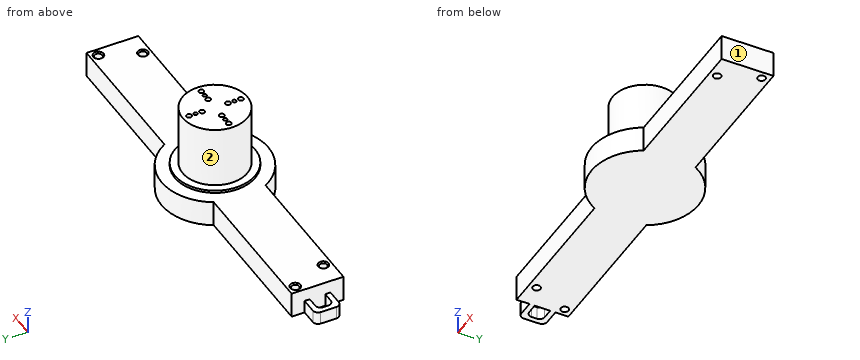
from build123d import *

# Parameters (mm, degrees)
SZKIC1_W                    = 150
SZKIC1_H                    = 20
DODANIE_WYCI_GNI_CIE1_DEPTH = 10
SZKIC2_R                    = 20.61119484
DODANIE_WYCI_GNI_CIE2_DEPTH = 10
SZKIC3_R                    = 12.5
DODANIE_WYCI_GNI_CIE5_DEPTH = 25
SZKIC8_R                    = 15.5
DODANIE_WYCI_GNI_CIE6_DEPTH = 1
SZKIC9_R                    = 1.5
WYTNIJ_WYCI_GNI_CIE1_DEPTH  = 10
SFAZOWANIE1_SIZE            = 0.5
SZKIC10_W                   = 5
SZKIC10_H                   = 10
DODANIE_WYCI_GNI_CIE7_DEPTH = 8
SZKIC11_W                   = 6
SZKIC11_H                   = 6
WYTNIJ_WYCI_GNI_CIE2_DEPTH  = 8
ZAOKR_GLENIE1_R             = 2
SZKIC12_R                   = 1
SZKIC12_R_2                 = 0.75
WYTNIJ_WYCI_GNI_CIE3_DEPTH  = 5


with BuildPart() as part:
    # Szkic1 → Dodanie-wyciągnięcie1 (new body)
    with BuildSketch(Plane.XY):
        Rectangle(SZKIC1_W, SZKIC1_H)
    extrude(amount=DODANIE_WYCI_GNI_CIE1_DEPTH)

    # Szkic2 → Dodanie-wyciągnięcie2 (add)
    with BuildSketch(Plane.XY.offset(10)):
        Circle(SZKIC2_R)
    extrude(amount=-DODANIE_WYCI_GNI_CIE2_DEPTH)

    # Szkic3 → Dodanie-wyciągnięcie5 (add)
    with BuildSketch(Plane.XY.offset(10)):
        Circle(SZKIC3_R)
    extrude(amount=DODANIE_WYCI_GNI_CIE5_DEPTH)

    # Szkic8 → Dodanie-wyciągnięcie6 (add)
    with BuildSketch(Plane.XY.offset(10)):
        Circle(SZKIC8_R)
    extrude(amount=DODANIE_WYCI_GNI_CIE6_DEPTH)

    # Szkic9 → Wytnij-wyciągnięcie1 (cut)
    with BuildSketch(Plane(origin=(0, 0, 0), x_dir=(-1, 0, 0), z_dir=(0, 0, -1))):
        with Locations((-72, 7)):
            Circle(SZKIC9_R)
        with Locations((-66, -7)):
            Circle(SZKIC9_R)
        with Locations((66, -7)):
            Circle(SZKIC9_R)
        with Locations((72, 7)):
            Circle(SZKIC9_R)
    extrude(amount=-WYTNIJ_WYCI_GNI_CIE1_DEPTH, mode=Mode.SUBTRACT)

    # Sfazowanie1
    sfazowanie1_edges = [part.edges().sort_by_distance(p)[0] for p in [
        (73.5, 7, 10),
        (67.5, -7, 10),
        (-64.5, -7, 10),
        (-70.5, 7, 10),
    ]]
    chamfer(sfazowanie1_edges, length=SFAZOWANIE1_SIZE)

    # Szkic10 → Dodanie-wyciągnięcie7 (add)
    with BuildSketch(Plane.ZY.offset(75)):
        with Locations((2.5, 0)):
            Rectangle(SZKIC10_W, SZKIC10_H)
    extrude(amount=DODANIE_WYCI_GNI_CIE7_DEPTH)

    # Szkic11 → Wytnij-wyciągnięcie2 (cut)
    with BuildSketch(Plane(origin=(0, 0, 0), x_dir=(-1, 0, 0), z_dir=(0, 0, -1))):
        with Locations((78, 0)):
            Rectangle(SZKIC11_W, SZKIC11_H)
    extrude(amount=-WYTNIJ_WYCI_GNI_CIE2_DEPTH, mode=Mode.SUBTRACT)

    # Zaokrąglenie1
    zaokr_glenie1_edges = [part.edges().sort_by_distance(p)[0] for p in [
        (-81, 3, 2.5),
        (-81, -3, 2.5),
        (-83, -5, 2.5),
        (-83, 5, 2.5),
    ]]
    fillet(zaokr_glenie1_edges, radius=ZAOKR_GLENIE1_R)

    # Szkic12 → Wytnij-wyciągnięcie3 (cut)
    with BuildSketch(Plane.XY.offset(35)):
        with Locations((-5, 0)):
            Circle(SZKIC12_R)
        with Locations((-10, 0)):
            Circle(SZKIC12_R)
        with Locations((0, 10)):
            Circle(SZKIC12_R)
        with Locations((0, 5)):
            Circle(SZKIC12_R)
        with Locations((10, 0)):
            Circle(SZKIC12_R)
        with Locations((5, 0)):
            Circle(SZKIC12_R)
        with Locations((0, -10)):
            Circle(SZKIC12_R)
        with Locations((0, -5)):
            Circle(SZKIC12_R)
        with Locations((-7.5, 0)):
            Circle(SZKIC12_R_2)
        with Locations((0, 7.5)):
            Circle(SZKIC12_R_2)
        with Locations((7.5, 0)):
            Circle(SZKIC12_R_2)
        with Locations((0, -7.5)):
            Circle(SZKIC12_R_2)
    extrude(amount=-WYTNIJ_WYCI_GNI_CIE3_DEPTH, mode=Mode.SUBTRACT)


solid = part.part
Input: part model. Units: mm. Frame: model coordinates. Face numbers are marked on the shaded views. A direction names the side the tool comes from. Give positions to 0.01 mm unless a question says otherwise; leave off trailing zeros. Loops run counter-clockwise (first coordinate to the right, second up) from the corner with the lowest first, then second, coordinate; pieces in that order, holes last. Notation, with made-up numbers: (-18.75, 1.5) -> (24.25, 1.5) arc R31 cw to (24.25, 31.5) -> close; hole circle Ø5 at (-13, 58). An arc over 180 degrees is marked (long way). Answer as a JSON object with one key per item and string values. Group by question number.
Item 1: Pin query (flat end, axial travel): P1, Ø0.6, axis at x = -5, y = 0.5, coming from the +Z side; P2, Ø4.5, axis at x = -78, z = 1.5, coming from the -Y side; P3, Ø11, axis at x = -48.5, z = 7.5, coming from the +Y side. Return the tip coordinate at first contact, or that it passes through.
Item 2: Line query: probe 1 along Y at (x, z) = (66, 5); probe 2 along Z at (x, y) = (-49, 4.5); probe 3 along Y at (x, z) = (64, 9). Output: solid intervals per line, ascending.
Item 3: Reachability of the marked faces 1 and 2 from +Z, -Z, +X, -X, +Y, -Y: full face, straight path, thin tool, end or side. Return the list, or none.
Item 4: Cut plane B-B, the plane z = 27. Return the cut outline in (x, y), and give its area (3 significant figures).
Item 5: Cut plane A-A, the plane x = -61.5. Return the cut outline in (y, z), and give its area (3 significant figures).
Checks:
{
 "1": {"P1": "stops at z = 30", "P2": "stops at y = -5", "P3": "stops at y = 10"},
 "2": {"probe 1": "y = -10 to -8.5, -5.5 to 10", "probe 2": "z = 0 to 10", "probe 3": "y = -10 to 10"},
 "3": {"face 1": "+Z, -Z, +X, +Y, -Y", "face 2": "+Z"},
 "4": {"outline": "circle Ø25 at (0, 0)", "area": "491 mm²"},
 "5": {"outline": "(-10, 0) -> (10, 0) -> (10, 10) -> (-10, 10) -> close", "area": "200 mm²"}
}
